Autodesk Inventor part; units mm, degrees
ref_plane "YZ Plane" through (0, 0, 0) normal (1, 0, 0) x (0, 1, 0)
ref_plane "XZ Plane" through (0, 0, 0) normal (0, 1, 0) x (-1, 0, 0)
ref_plane "XY Plane" through (0, 0, 0) normal (0, 0, 1) x (1, 0, 0)
sketch "Эскиз1" plane through (0, 0, 0) normal (0, 1, 0) x (-1, 0, 0)
  circle A0 centre (0, 0) radius 5
  circle A1 centre (0, 0) radius 25
  circle A2 centre (14, 0) radius 6.1
  circle A3 centre (4.3262, 13.3148) radius 6.1
  circle A4 centre (-11.3262, 8.229) radius 6.1
  circle A5 centre (-11.3262, -8.229) radius 6.1
  circle A6 centre (4.3262, -13.3148) radius 6.1
  dimension "d2" = 10
  dimension "d3" = 50
  dimension "d4" = 12.2
  dimension "d5" = 14
  dimension "d6" = 360
extrude "Выдавливание1" add sketch "Эскиз1" along normal blind 10
properties part number "ротор редуктора"
The listing builds one solid part. Answer for the finished solid, in the listing's coordinates (mm). Give positions to 0.01 mm unless a question says otherwise; leave off trailing zeros. Loops run counter-clockwise (first coordinate to the right, second up) from the corner with the lowest first, then second, coordinate; pieces in that order, holes last. Notation, with made-up numbers: (26.25, -23) - (85.25, -23) arc R17 cw to (85.25, 4) - close; hole circle Ø9 at (25.25, 88.5). An arc over 180 degrees is marked (long way). Answer as CSV lines item,"result". Start each with the question number.
Item 1: A cutting plane is placed at A-A on z = 0. Determine the outline of the cut face in (x, y), then the cut area to 3 significant figures.
Item 2: A cutting plane is placed at C-C on y = 7.5. Determine the outline of the cut face in (x, z), then the cut area to 3 significant figures.
Item 3: Each of these flat-tipped pins is pushed along its axis until it touches: pin 1 (5 mm diameter, centred on x = 0.5, z = 11.5, fed in from -Y); pin 2 (6 mm diameter, centred on x = 0, z = 0, fed in from +Y); pin 3 (4 mm diameter, centred on y = 8, z = 16.5, fed in from -X); pin 4 (2 mm diameter, centred on x = 14, y = 5, fed in from -Z). Where does it stop, or does it pass through?
Item 4: The mould has two halves that part along X. Classify faces 1 (the face through (0.3, 10, -5.2)), 2 (the face through (12.649, 4.93, -2.274)), 3 (the face through (-23.846, 4.93, -7.509)): +X half, -X half, draft (parallel to the pull), parting line (faces both ways), or undercut.
Item 5: A cutting plane is placed at D-D on x = 7. Determine the outline of the cut face in (y, z), then the cut area to 3 significant figures.
Item 6: A cutting plane is placed at B-B on x = 0. Determine the outline of the cut face in (y, z), then the cut area to 3 significant figures.
Item 7: Find the intervals of material crossed by line 1 (Z direction, x = -1, y = 5); line 2 (Z direction, x = 9, y = 5.25); line 3 (Z direction, x = -0.5, y = 7.5) (3 decimals), in increasing order. Write a range as from..to.
Found:
1,outline,"(-25, 0) - (-20.1, 0) - (-20.1, 10) - (-25, 10) - close; (-7.9, 0) - (-5, 0) - (-5, 10) - (-7.9, 10) - close; (5, 0) - (25, 0) - (25, 10) - (5, 10) - close"
1,area,"278 mm^2"
2,outline,"circle Ø50 at (0, 0); hole circle Ø12.2 at (-14, 0); hole circle Ø12.2 at (-4.33, -13.31); hole circle Ø12.2 at (-4.33, 13.31); hole circle Ø10 at (0, 0); hole circle Ø12.2 at (11.33, -8.23); hole circle Ø12.2 at (11.33, 8.23)"
2,area,"1,300 mm^2"
3,pin 1,"stops at y = 0"
3,pin 2,"passes through"
3,pin 3,"stops at x = -20.37"
3,pin 4,"stops at z = -21.35"
4,face 1,"draft"
4,face 2,"undercut"
4,face 3,"parting line"
5,outline,"(0, -24) - (10, -24) - (10, -12.53) - (0, -12.53) - close; (0, -3.93) - (10, -3.93) - (10, 3.93) - (0, 3.93) - close; (0, 12.53) - (10, 12.53) - (10, 24) - (0, 24) - close"
5,area,"308 mm^2"
6,outline,"(0, -25) - (10, -25) - (10, -17.62) - (0, -17.62) - close; (0, -9.01) - (10, -9.01) - (10, -5) - (0, -5) - close; (0, 5) - (10, 5) - (10, 9.01) - (0, 9.01) - close; (0, 17.62) - (10, 17.62) - (10, 25) - (0, 25) - close"
6,area,"228 mm^2"
7,line 1,"z = -24.98..-18.43, -8.2..-4.9, 4.9..8.2, 18.43..24.98"
7,line 2,"z = -23.32..-13.87, -2.59..2.59, 13.87..23.32"
7,line 3,"z = -24.995..-18.066, -8.564..-4.975, 4.975..8.564, 18.066..24.995"
